Model file for the job. Use its own axes, mm. A direction names the side the tool comes from. Coordinates: 2 decimals unless noted, no trailing zeros. Loops run counter-clockwise (first coordinate to the right, second up) from the corner with the lowest first, then second, coordinate; pieces in that order, holes last.
from build123d import *

# Parameters (mm, degrees)
F0_R           = 5.5025
F1_DEPTH       = 1.26
F2_R           = 5.03
F3_DEPTH       = 0.38
F4_R           = 2.75
F5_DEPTH       = 0.26
F7_DEPTH       = 7.5
F9_DEPTH       = 0.26
F10_R          = 0.26
F13_DEPTH      = 2.3
F14_R          = 0.765
F15_DEPTH      = 0.38
F16_R          = 0.515
F17_DEPTH      = 10.6835
F18_DEPTH      = 1.5
F19_F1_R       = 0.26
F19_F2_R       = 0.26
F21_DEPTH      = 15
F23_END_RADIUS = 5.5025
F23_REACH      = 10.1867902517
F25_DEPTH      = 10


# Not quite as in the source:
# - after a boolean that leaves OpenCascade's solid faulty, fix() repairs it


with BuildPart() as f1:
    # F0 (on Front) → F1 (new body)
    with BuildSketch(Plane.XZ):
        Circle(F0_R)
    extrude(amount=F1_DEPTH)

    # F2 (on face) → F3 (cut)
    with BuildSketch(Plane(origin=(0, 0, 0), x_dir=(-1, 0, 0), z_dir=(0, 1, 0))):
        Circle(F2_R)
    extrude(amount=-F3_DEPTH, mode=Mode.SUBTRACT)

    # F4 (on face) → F5 (cut)
    with BuildSketch(Plane(origin=(0, -0.38, 0), x_dir=(-1, 0, 0), z_dir=(0, 1, 0))):
        Circle(F4_R)
    extrude(amount=-F5_DEPTH, mode=Mode.SUBTRACT)

    # F6 (on face) → F7 (cut, symmetric)
    with BuildSketch(Plane.XZ.offset(1.26)):
        with BuildLine():
            ThreePointArc((-1.1142352941, 3.6852380804), (0, 3.85), (1.1142352941, 3.6852380804))
            ThreePointArc((1.1142352941, 3.6852380804), (1.6128818785, 3.952355253), (1.3457647059, 4.4510018374))
            ThreePointArc((1.3457647059, 4.4510018374), (0, 4.65), (-1.3457647059, 4.4510018374))
            ThreePointArc((-1.3457647059, 4.4510018374), (-1.6128818785, 3.952355253), (-1.1142352941, 3.6852380804))
        make_face()
        with BuildLine():
            ThreePointArc((1.1142352941, -3.6852380804), (0, -3.85), (-1.1142352941, -3.6852380804))
            ThreePointArc((-1.1142352941, -3.6852380804), (-1.6128818785, -3.952355253), (-1.3457647059, -4.4510018374))
            ThreePointArc((-1.3457647059, -4.4510018374), (0, -4.65), (1.3457647059, -4.4510018374))
            ThreePointArc((1.3457647059, -4.4510018374), (1.6128818785, -3.952355253), (1.1142352941, -3.6852380804))
        make_face()
    extrude(amount=F7_DEPTH, both=True, mode=Mode.SUBTRACT)

    # F8 (on face) → F9 (cut)
    with BuildSketch(Plane.XZ.offset(1.26)):
        with BuildLine():
            Line((-2, -2.38), (-2, 2.38))
            Line((-2, 2.38), (-3.5, 2.38))
            Line((-3.5, 2.38), (-3.5, 1.479089023))
            ThreePointArc((-3.5, 1.479089023), (-3.468035085, 1.354189063), (-3.38, 1.26))
            ThreePointArc((-3.38, 1.26), (-3.291964915, 1.165810937), (-3.26, 1.040910977))
            Line((-3.26, 1.040910977), (-3.26, -1.040910977))
            ThreePointArc((-3.26, -1.040910977), (-3.291964915, -1.165810937), (-3.38, -1.26))
            ThreePointArc((-3.38, -1.26), (-3.468035085, -1.354189063), (-3.5, -1.479089023))
            Line((-3.5, -1.479089023), (-3.5, -2.38))
            Line((-3.5, -2.38), (-2, -2.38))
        make_face()
    extrude(amount=-F9_DEPTH, mode=Mode.SUBTRACT)

    # F10
    f10_edges = [f1.edges().sort_by_distance(p)[0] for p in [
        (-2, -1.13, 2.38),
        (-3.5, -1.13, 2.38),
        (-3.5, -1.13, -2.38),
        (-2, -1.13, -2.38),
    ]]
    fillet(f10_edges, radius=F10_R)

    # F12 (on offset) → F13 (join, through all)
    with BuildSketch(Plane.YZ.offset(-5.56)):
        with BuildLine():
            Line((-1, -1.26), (-1, 1.26))
            Line((-1, 1.26), (-2, 1.26))
            ThreePointArc((-2, 1.26), (-3.26, 0), (-2, -1.26))
            Line((-2, -1.26), (-1, -1.26))
        make_face()
    extrude(amount=F13_DEPTH)

    # F14 (on face) → F15 (cut)
    with BuildSketch(Plane(origin=(-5.56, 0, 0), x_dir=(0, -1, 0), z_dir=(-1, 0, 0))):
        with Locations((2, 0)):
            Circle(F14_R)
    extrude(amount=-F15_DEPTH, mode=Mode.SUBTRACT)

    # F16 (on face) → F17 (cut, through all)
    with BuildSketch(Plane(origin=(-5.18, 0, 0), x_dir=(0, -1, 0), z_dir=(-1, 0, 0))):
        with Locations((2, 0)):
            Circle(F16_R)
    extrude(amount=-F17_DEPTH, mode=Mode.SUBTRACT)

    # F18 (cut): a face of the model
    f18_faces = [f1.faces().sort_by_distance(p)[0] for p in [
        (-2.6893148123, -1, 0),
    ]]
    extrude(f18_faces, amount=F18_DEPTH, mode=Mode.SUBTRACT)

    # F19: fillet of radius 0.26 on 4 edges, made by hand

    # F19_f1
    f19_f1_edges = [f1.edges().sort_by_distance(p)[0] for p in [
        (-5.4581479725, -1, 1.26),
        (-5.4581479725, -1, -1.26),
    ]]
    fillet(f19_f1_edges, radius=F19_F1_R)

    # F19_f2
    f19_f2_edges = [f1.edges().sort_by_distance(p)[0] for p in [
        (-4.3681479725, -1.26, 1.26),
        (-4.3681479725, -1.26, -1.26),
    ]]
    fillet(f19_f2_edges, radius=F19_F2_R)

    # F20 (on face) → F21 (cut)
    with BuildSketch(Plane.XZ.offset(1)):
        with BuildLine():
            ThreePointArc((-2.26, -2.38), (-2.0761522369, -2.3038477631), (-2, -2.12))
            Line((-2, -2.12), (-2, 2.12))
            ThreePointArc((-2, 2.12), (-2.0761522369, 2.3038477631), (-2.26, 2.38))
            Line((-2.26, 2.38), (-3.24, 2.38))
            ThreePointArc((-3.24, 2.38), (-3.4238477631, 2.3038477631), (-3.5, 2.12))
            Line((-3.5, 2.12), (-3.5, 1.479089023))
            ThreePointArc((-3.5, 1.479089023), (-3.468035085, 1.354189063), (-3.38, 1.26))
            ThreePointArc((-3.38, 1.26), (-3.2919649151, 1.165810937), (-3.2600000001, 1.0409109771))
            Line((-3.2600000001, 1.0409109771), (-3.2599999999, -1.0409109769))
            ThreePointArc((-3.2599999999, -1.0409109769), (-3.2919649149, -1.1658109369), (-3.38, -1.26))
            ThreePointArc((-3.38, -1.26), (-3.468035085, -1.354189063), (-3.5, -1.479089023))
            Line((-3.5, -1.479089023), (-3.5, -2.12))
            ThreePointArc((-3.5, -2.12), (-3.4238477631, -2.3038477631), (-3.24, -2.38))
            Line((-3.24, -2.38), (-2.26, -2.38))
        make_face()
    extrude(amount=F21_DEPTH, mode=Mode.SUBTRACT)

    f23_end = (Plane.ZX.offset(-0.76) * Cylinder(F23_END_RADIUS, 52.2556470224, mode=Mode.PRIVATE)).faces().sort_by_distance((-5.5025, -0.76, 0))[0]
    # F22 (on face) → F23 (join, up to the whole of a round face its end follows)
    with BuildSketch(Plane(origin=(-2, 0, 0), x_dir=(0, -1, 0), z_dir=(-1, 0, 0))):
        with BuildLine():
            Line((2.5, 2.75), (1.51, 3.3215767665))
            ThreePointArc((1.51, 3.3215767665), (1.3269872981, 3.5045894684), (1.26, 3.7545894684))
            Line((1.26, 3.7545894684), (1.26, 1.875))
            Line((1.26, 1.875), (1.26, 1.6671539031))
            ThreePointArc((1.26, 1.6671539031), (1.32, 1.7710769515), (1.44, 1.7710769515))
            Line((1.44, 1.7710769515), (2.1260254038, 1.375))
            Line((2.1260254038, 1.375), (2.5, 1.375))
            Line((2.5, 1.375), (2.5, 2.75))
        make_face()
        with BuildLine():
            ThreePointArc((1.26, -3.7545894684), (1.3269872981, -3.5045894684), (1.51, -3.3215767665))
            Line((1.51, -3.3215767665), (2.5, -2.75))
            Line((2.5, -2.75), (2.5, -1.375))
            Line((2.5, -1.375), (2.1260254038, -1.375))
            Line((2.1260254038, -1.375), (1.44, -1.7710769515))
            ThreePointArc((1.44, -1.7710769515), (1.32, -1.7710769515), (1.26, -1.6671539031))
            Line((1.26, -1.6671539031), (1.26, -1.875))
            Line((1.26, -1.875), (1.26, -3.7545894684))
        make_face()
    f23_long = extrude(amount=-F23_REACH, mode=Mode.PRIVATE)
    add(split(f23_long, bisect_by=f23_end, keep=Keep.BOTTOM, mode=Mode.PRIVATE))

    add(f1.part.fix(), mode=Mode.REPLACE)

    # F24 (on face) → F25 (cut)
    with BuildSketch(Plane(origin=(0, -0.38, 0), x_dir=(-1, 0, 0), z_dir=(0, 1, 0))):
        with BuildLine():
            ThreePointArc((-1.1142352941, -3.6852380804), (-1.6128818785, -3.952355253), (-1.3457647059, -4.4510018374))
            ThreePointArc((-1.3457647059, -4.4510018374), (0, -4.65), (1.3457647059, -4.4510018374))
            ThreePointArc((1.3457647059, -4.4510018374), (1.6128818785, -3.952355253), (1.1142352941, -3.6852380804))
            ThreePointArc((1.1142352941, -3.6852380804), (0, -3.85), (-1.1142352941, -3.6852380804))
        make_face()
        with BuildLine():
            ThreePointArc((-1.1142352941, 3.6852380804), (0, 3.85), (1.1142352941, 3.6852380804))
            ThreePointArc((1.1142352941, 3.6852380804), (1.6128818785, 3.952355253), (1.3457647059, 4.4510018374))
            ThreePointArc((1.3457647059, 4.4510018374), (0, 4.65), (-1.3457647059, 4.4510018374))
            ThreePointArc((-1.3457647059, 4.4510018374), (-1.6128818785, 3.952355253), (-1.1142352941, 3.6852380804))
        make_face()
    extrude(amount=-F25_DEPTH, mode=Mode.SUBTRACT)


solid = f1.part
Q1. Drill centre lines: line 1 (Z direction, x = -5.25, y = -2) (3 decimals); line 2 (X direction, y = -1.2, z = 0); line 3 (Z direction, x = 0, y = -0.25). Where is each one in solid material? Low to high.
Answers:
line 1: z = -1.26 to -0.765, 0.765 to 1.26
line 2: x = -5.56 to -3.26, -2 to 5.5
line 3: z = -5.5 to -5.03, 5.03 to 5.5
Q2. Flat gauge pins, fed straight in: P1, Ø1.2, axis at x = -3, z = -1, coming from the -Y side; P2, Ø0.8, axis at x = -4.5, y = -1.5, coming from the +Z side; P3, Ø1, axis at x = -2, y = -1, coming from the +Z side. Where does each tip first touch, or does it go through?
Answers:
P1: stops at y = -3.17
P2: stops at z = 3.58
P3: stops at z = 5.29
Q3. Slice it at B-B (x = 0). Count the separate pieces of the cut face and the enclosed holes in it, and give its area (3 significant figures).
Answers:
separate pieces: 3
enclosed holes: 0
area: 11.1 mm2
Q4. Slice it at C-C (z = -4.25). List the corners of the cut face in (x, y) (3 decimals), and give its area (3 significant figures).
Answers:
outline: (-3.495, -1.26) - (-1.586, -1.26) - (-1.586, -0.38) - (-2.69, -0.38) - (-2.69, 0) - (-3.495, 0) - close; (1.586, -1.26) - (3.495, -1.26) - (3.495, 0) - (2.69, 0) - (2.69, -0.38) - (1.586, -0.38) - close
area: 3.97 mm2
Q5. Which spindle directions (+Z, -Z, +X, -X, +Y, -Y) get a long thin tool onto all of the face, cutting with end or side? Do faces 4 (the cylindrical face through (0.02, -0.81, 4.65)), 5 (the flat face through (2, -1.26, 0)), 6 (the cylindrical face through (-5.373, -1.236, 0.034)), 7 (the flat face through (0, -0.64, 0)), 8 (the flat face through (-3.26, -3, 0)). Say none if no direction does.
Answers:
face 4: +Y, -Y
face 5: +X
face 6: -X
face 7: +Y
face 8: -Y
Q6. Mould opens along X. For faces 1 (the cylindrical face through (0.655, -0.187, 4.987)), 2 (the cylindrical face through (-4.233, -1.485, 0.023)), 3 (the flat face through (-5.56, -2, 1)) say: +X half, -X half, draft (parallel to the pull), parting line (faces both ways), or undercut.
Answers:
face 1: undercut
face 2: draft
face 3: -X half
